Part print with two shaded views. Sizes in mm from the minimum x, y, z corner. Coordinates: 2 decimals unless noted, no trailing zeros. Loops run counter-clockwise (first coordinate to the right, second up) from the corner with the lowest first, then second, coordinate; pieces in that order, holes last.
(1) Slice it at B-B (z = 12.7). Give the cut face in (x, y), and give its area (3 significant figures).
(2) Slice it at A-A (z = 25.4). Give the cut face in (x, y) (3 decimals), and give its area (3 significant figures).
(3) Slice it at D-D (y = 9). Give the cut face in (x, z).
(4) Flat gauge pin, fed straight in: P1, Ø4, axis at x = 6, z = 7.5, coming from the -Y side. Where does the tip first touch, or does it go through?
(5) Slice it at C-C (x = 9.5). Give the cut face in (y, z) (3 decimals).
(6) Wall check: L1, parallel to Y at x = 8, z = 38; L2, parallel to Z at x = 6.25, y = 70.5; L3, parallel to Y at x = 8.75, z = 21 (3 decimals). Give the ranges that are in metal, low to high.
(7) Two-plate mould, pull along Z, no slides. Class the marked faces 1, 2, 3 and 4: pulls with the +Z half, pulls with the -Z half, needs draft (parallel to the pull), parting line crosses it, or undercut.
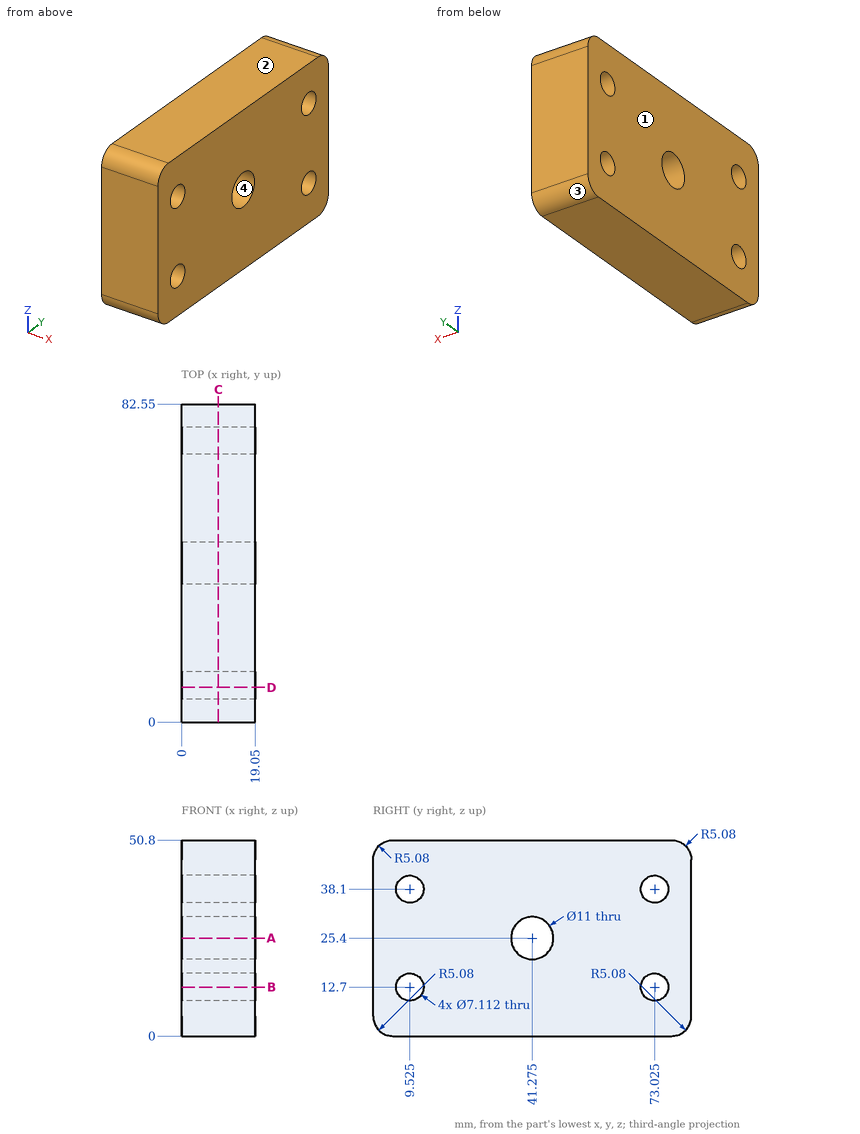
Response values:
1. outline: (0, 0) - (19.05, 0) - (19.05, 5.97) - (0, 5.97) - close; (0, 13.08) - (19.05, 13.08) - (19.05, 69.47) - (0, 69.47) - close; (0, 76.58) - (19.05, 76.58) - (19.05, 82.55) - (0, 82.55) - close
1. area: 1,300 mm2
2. outline: (0, 0) - (19.05, 0) - (19.05, 35.775) - (0, 35.775) - close; (0, 46.775) - (19.05, 46.775) - (19.05, 82.55) - (0, 82.55) - close
2. area: 1,360 mm2
3. outline: (0, 0) - (19.05, 0) - (19.05, 9.18) - (0, 9.18) - close; (0, 16.22) - (19.05, 16.22) - (19.05, 34.58) - (0, 34.58) - close; (0, 41.62) - (19.05, 41.62) - (19.05, 50.8) - (0, 50.8) - close
4. P1: stops at y = 0
5. outline: (0, 5.08) arc R5.08 ccw to (5.08, 0) - (77.47, 0) arc R5.08 ccw to (82.55, 5.08) - (82.55, 45.72) arc R5.08 ccw to (77.47, 50.8) - (5.08, 50.8) arc R5.08 ccw to (0, 45.72) - close; hole circle Ø7.112 at (9.525, 12.7); hole circle Ø7.112 at (9.525, 38.1); hole circle Ø11 at (41.275, 25.4); hole circle Ø7.112 at (73.025, 12.7); hole circle Ø7.112 at (73.025, 38.1)
6. L1: y = 0 to 5.97, 13.08 to 69.47, 76.58 to 82.55
6. L2: z = 0 to 10.2, 15.2 to 35.6, 40.6 to 50.8
6. L3: y = 0 to 37.975, 44.575 to 82.55
7. face 1: needs draft
7. face 2: pulls with the +Z half
7. face 3: pulls with the -Z half
7. face 4: undercut
